```python
from build123d import *

# Parameters (mm, degrees)
SKETCH1_R           = 1.6
BOSS_EXTRUDE1_DEPTH = 4.6
CUT_EXTRUDE2_DEPTH  = 1.4


with BuildPart() as part:
    # Sketch1 → Boss-Extrude1 (new body)
    with BuildSketch(Plane.XY):
        with BuildLine():
            Line((-11.319805153, 23.328427125), (-23.328427125, 11.319805153))
            ThreePointArc((-23.328427125, 11.319805153), (-24.19551813, 10.022111758), (-24.5, 8.491378029))
            Line((-24.5, 8.491378029), (-24.5, -8.491378029))
            ThreePointArc((-24.5, -8.491378029), (-24.19551813, -10.022111758), (-23.328427125, -11.319805153))
            Line((-23.328427125, -11.319805153), (-11.319805153, -23.328427125))
            ThreePointArc((-11.319805153, -23.328427125), (-10.022111758, -24.19551813), (-8.491378029, -24.5))
            Line((-8.491378029, -24.5), (8.491378029, -24.5))
            ThreePointArc((8.491378029, -24.5), (10.022111758, -24.19551813), (11.319805153, -23.328427125))
            Line((11.319805153, -23.328427125), (23.328427125, -11.319805153))
            ThreePointArc((23.328427125, -11.319805153), (24.19551813, -10.022111758), (24.5, -8.491378029))
            Line((24.5, -8.491378029), (24.5, 8.491378029))
            ThreePointArc((24.5, 8.491378029), (24.19551813, 10.022111758), (23.328427125, 11.319805153))
            Line((23.328427125, 11.319805153), (11.319805153, 23.328427125))
            ThreePointArc((11.319805153, 23.328427125), (10.022111758, 24.19551813), (8.491378029, 24.5))
            Line((8.491378029, 24.5), (-8.491378029, 24.5))
            ThreePointArc((-8.491378029, 24.5), (-10.022111758, 24.19551813), (-11.319805153, 23.328427125))
        make_face()
        with Locations((-4.949747468, 4.949747468)):
            Circle(SKETCH1_R, mode=Mode.SUBTRACT)
        with Locations((4.949747468, 4.949747468)):
            Circle(SKETCH1_R, mode=Mode.SUBTRACT)
        with Locations((4.949747468, -4.949747468)):
            Circle(SKETCH1_R, mode=Mode.SUBTRACT)
        with Locations((-4.949747468, -4.949747468)):
            Circle(SKETCH1_R, mode=Mode.SUBTRACT)
    extrude(amount=BOSS_EXTRUDE1_DEPTH)

    # Sketch3 → Cut-Extrude2 (cut)
    with BuildSketch(Plane.XY.offset(4.6)):
        with BuildLine():
            Line((8.491378029, 22), (-8.491378029, 22))
            ThreePointArc((-8.491378029, 22), (-9.027134834, 21.893431346), (-9.481327522, 21.589949494))
            Line((-9.481327522, 21.589949494), (-21.489949494, 9.581327522))
            ThreePointArc((-21.489949494, 9.581327522), (-21.793431346, 9.127134834), (-21.9, 8.591378029))
            Line((-21.9, 8.591378029), (-21.9, -8.391378029))
            ThreePointArc((-21.9, -8.391378029), (-21.793431346, -8.927134834), (-21.489949494, -9.381327522))
            Line((-21.489949494, -9.381327522), (-9.481327522, -21.389949494))
            ThreePointArc((-9.481327522, -21.389949494), (-9.027134834, -21.693431346), (-8.491378029, -21.8))
            Line((-8.491378029, -21.8), (8.491378029, -21.8))
            ThreePointArc((8.491378029, -21.8), (9.027134834, -21.693431346), (9.481327522, -21.389949494))
            Line((9.481327522, -21.389949494), (21.489949494, -9.381327522))
            ThreePointArc((21.489949494, -9.381327522), (21.793431346, -8.927134834), (21.9, -8.391378029))
            Line((21.9, -8.391378029), (21.9, 8.591378029))
            ThreePointArc((21.9, 8.591378029), (21.793431346, 9.127134834), (21.489949494, 9.581327522))
            Line((21.489949494, 9.581327522), (9.481327522, 21.589949494))
            ThreePointArc((9.481327522, 21.589949494), (9.027134834, 21.893431346), (8.491378029, 22))
        make_face()
    extrude(amount=-CUT_EXTRUDE2_DEPTH, mode=Mode.SUBTRACT)


solid = part.part
```
Geometry check sheet. Reference: the model listing, model coordinates, mm. A direction names the side the tool comes from. Round coordinates to 2 decimals unless told otherwise and drop trailing zeros. Order: outer loops, then holes, each group sorted by start corner. A loop starts at its lowest first (then second) coordinate and runs counter-clockwise, first axis right, second up. Notation, with made-up numbers: (10.5, -25) - (30.5, -25) arc R29 cw to (30.5, 11) - close; hole circle Ø1 at (70.25, 14). An arc over 180 degrees is marked (long way). Use a Markdown table: item, result. Add a question column.
(1) Material ranges on line 1 along Y through (x, z) = (-4, 4); line 2 along X through (y, z) = (4, 3.85); line 3 along Y through (x, z) = (-6, 0.85), recorded low to high. Write a range as [from, to].
(2) Release check for a two-part mould opening along X. For faces 1 (the flat face through (0, -24.5, 2)), 2 (the cylindrical face through (-4.09, -3.6, 1.58)), 3 (the cylindrical face through (24.204, 10.002, 2.268)) record: pulls with the +X half, pulls with the -X half, needs draft (parallel to the pull), parting line crosses it, or undercut.
(3) Sectioned sample at A-A, the plane y = 1. Enter the section's corners in (x, z).
(4) Tool access check on faces 4 (the flat face through (17.24, -17.41, 2.27)), 5 (the flat face through (15.57, 15.5, 3.91)). Record the directions out of +Z, -Z, +X, -X, +Y, -Y that give a thin tool (end or side, any length) a straight path to the whole face; none if there is none.
(5) Sectioned sample at B-B, the plane x = -7.5. Enter the section's corners in (y, z), and give its area (3 significant figures).
(6) Sectioned sample at C-C, the plane z = 0.9. Enter the section's corners in (x, y).
(7) Depth check by flat-ended pin: pin 1 (4 mm diameter, centred on x = -4.95, y = -4.95, fed in from +Z). Enter the tip coordinate at first touch or a pass-through.
Answers below:
| question | item | result |
|---|---|---|
| 1 | line 1 | [-24.5, -21.8], [22, 24.5] |
| 1 | line 2 | [-24.5, -21.9], [21.9, 24.5] |
| 1 | line 3 | [-24.5, -6.16], [-3.74, 3.74], [6.16, 24.5] |
| 2 | face 1 | needs draft |
| 2 | face 2 | undercut |
| 2 | face 3 | pulls with the +X half |
| 3 | outline | (-24.5, 0) - (24.5, 0) - (24.5, 4.6) - (21.9, 4.6) - (21.9, 3.2) - (-21.9, 3.2) - (-21.9, 4.6) - (-24.5, 4.6) - close |
| 4 | face 4 | +Z, -Z, +X, -Y |
| 4 | face 5 | +Z |
| 5 | outline | (-24.5, 0) - (24.5, 0) - (24.5, 4.6) - (22, 4.6) - (22, 3.2) - (-21.8, 3.2) - (-21.8, 4.6) - (-24.5, 4.6) - close |
| 5 | area | 164 mm² |
| 6 | outline | (-24.5, -8.49) arc R4 ccw to (-23.33, -11.32) - (-11.32, -23.33) arc R4 ccw to (-8.49, -24.5) - (8.49, -24.5) arc R4 ccw to (11.32, -23.33) - (23.33, -11.32) arc R4 ccw to (24.5, -8.49) - (24.5, 8.49) arc R4 ccw to (23.33, 11.32) - (11.32, 23.33) arc R4 ccw to (8.49, 24.5) - (-8.49, 24.5) arc R4 ccw to (-11.32, 23.33) - (-23.33, 11.32) arc R4 ccw to (-24.5, 8.49) - close; hole circle Ø3.2 at (-4.95, -4.95); hole circle Ø3.2 at (-4.95, 4.95); hole circle Ø3.2 at (4.95, -4.95); hole circle Ø3.2 at (4.95, 4.95) |
| 7 | pin 1 | z = 3.2 |
